Autodesk Inventor part; units mm, degrees
ref_plane "Work Plane1" through (0, 0, 0) normal (0, 0, 1) x (1, 0, 0)
ref_plane "YZ Plane" through (0, 0, 0) normal (1, 0, 0) x (0, 1, 0)
ref_plane "XZ Plane" through (0, 0, 0) normal (0, 1, 0) x (-1, 0, 0)
ref_plane "Work Plane1" through (0, 0, 0) normal (0, 0, 1) x (1, 0, 0)
sketch "Sketch1" plane through (0, 0, 0) normal (0, 0, 1) x (1, 0, 0)
  circle A0 centre (0, 0) radius 14
  circle A1 centre (0, 0) radius 10
  line L0 (0, -14) -> (0, 14)
  point P0 (0, 10)
  point P1 (0, -10)
  dimension "d1" = 4
  dimension "d4" = 20
extrude "Extrusion1" add sketch "Sketch1" along normal mid plane 4 contours L0 A1 A0 picked at (-1.9145, -12.4342)
chamfer "Chamfer1" distance 3.175 angle 45 1 edges at (0, 14, 0)
properties part number "2101b_Tx_Coil_Spacer_short_v1" material "Acetal Resin, White"
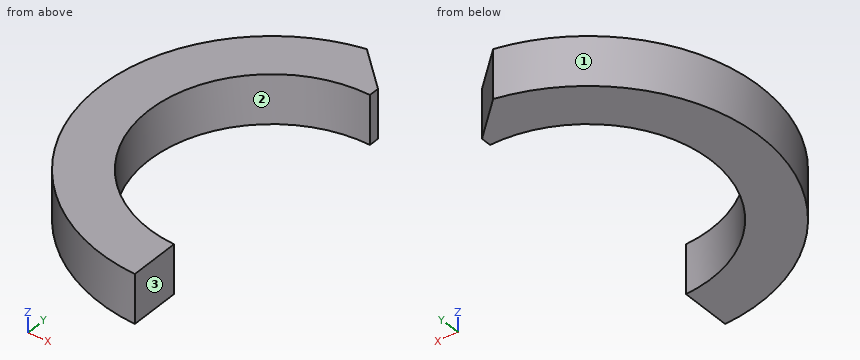
Verification items for the finished model (mm, model axes). Face numbers are marked on the shaded views. Coordinates: 2 decimals unless noted, no trailing zeros. Loops run counter-clockwise (first coordinate to the right, second up) from the corner with the lowest first, then second, coordinate; pieces in that order, holes last. Notation, with made-up numbers: (-39.5, 0) - (-10.5, 0) arc R30 ccw to (-10.5, 32) - close; hole circle Ø2 at (-7.75, 3). An arc over 180 degrees is marked (long way). Put each result on its own line as item: value.
Item 1: Section check A-A (x = -9.5). Enter the section's corners in (y, z), then the cut area to 3 significant figures.
Conclusion:
outline: (-10.28, -2) - (-3.12, -2) - (-3.12, 2) - (-10.28, 2) - close; (3.12, -2) - (10.28, -2) - (10.28, 2) - (3.12, 2) - close
area: 57.3 mm2
Item 2: Section check C-C (y = 8.5). Enter the section's corners in (x, z).
Conclusion:
outline: (-11.12, -2) - (-5.27, -2) - (-5.27, 2) - (-11.12, 2) - close
Item 3: Scan lines: line 1 along Y through (x, z) = (-1, 0.75); line 2 along Y through (x, z) = (-4.75, 0.8); line 3 along X through (y, z) = (-3.5, -1.8). Record each from-to range of solid material in increasing order.
Conclusion:
line 1: y = -13.96 to -9.95, 9.95 to 11.72
line 2: y = -13.17 to -8.8, 8.8 to 13.17
line 3: x = -13.56 to -9.37
Item 4: Section check B-B (z = 1.4). Enter the section's corners in (x, y) (3 decimals), then the cut area to 3 significant figures.
Conclusion:
outline: (-3.155, 13.64) arc R14 ccw to (0, -14) - (0, -10) arc R10 cw to (0, 10) - (0, 10.825) - close
area: 146 mm2
Item 5: Draft check along Y on the marked faces 1, 2 and 3. Enter one of: pulls with the +Y half, pulls with the -Y half, needs draft (parallel to the pull), parting line crosses it, or undercut.
Conclusion:
face 1: parting line crosses it
face 2: undercut
face 3: needs draft
Item 6: Section check D-D (x = -0.75). Enter the section's corners in (y, z), then the cut area to 3 significant figures.
Conclusion:
outline: (-13.98, -2) - (-9.97, -2) - (-9.97, 2) - (-13.98, 2) - close; (9.97, -2) - (11.49, -2) - (11.49, 2) - (9.97, 2) - close
area: 22.1 mm2
Item 7: Gauge pin test, flat ends, axial feed: pin 1 Ø1 at (y, z) = (-1.5, 0.5) entering from -X; pin 2 Ø1 at (x, z) = (-5, 1) entering from -Y. Record the tip position at first contact, or that the pin passes through.
Conclusion:
pin 1: stops at x = -13.96
pin 2: stops at y = -13.26
